Part model, mm, in its own coordinate system. A direction names the side the tool comes from. Round coordinates to 2 decimals unless told otherwise and drop trailing zeros. Loops run counter-clockwise (first coordinate to the right, second up) from the corner with the lowest first, then second, coordinate; pieces in that order, holes last.
from build123d import *

# Parameters (mm, degrees)
SKETCH_1_R      = 1
EXTRUDE_1_DEPTH = 1
SKETCH_1_3_W    = 1
SKETCH_1_3_H    = 4
EXTRUDE_2_DEPTH = 5
SKETCH_2_W      = 4
SKETCH_2_H      = 1
EXTRUDE_3_DEPTH = 2
FILLET_1_R      = 1
FILLET_2_R      = 2
FILLET_3_R      = 1


with BuildPart() as part:
    # 草圖1 → 填料-伸長1 (new body)
    with BuildSketch(Plane(origin=(0, 0, 0), x_dir=(1, 0, 0), z_dir=(0, 1, 0))):
        with BuildLine():
            ThreePointArc((0, -2), (2, 0), (0, 2))
            Line((0, 2), (-2, 2))
            Line((-2, 2), (-2, -2))
            Line((-2, -2), (0, -2))
        make_face()
        with Locations(Location((0, 0, 0), (0, 0, 270))):
            Circle(SKETCH_1_R, mode=Mode.SUBTRACT)
    extrude(amount=EXTRUDE_1_DEPTH)

    # 草圖1<3> → 填料-伸長2 (add)
    with BuildSketch(Plane(origin=(0, 0, 0), x_dir=(1, 0, 0), z_dir=(0, 1, 0))):
        with Locations((-2.5, 0)):
            Rectangle(SKETCH_1_3_W, SKETCH_1_3_H)
    extrude(amount=EXTRUDE_2_DEPTH)

    # 草圖2 → 填料-伸長3 (add)
    with BuildSketch(Plane(origin=(-2, 0, 0), x_dir=(0, 0, -1), z_dir=(1, 0, 0))):
        with Locations((0, 4.5)):
            Rectangle(SKETCH_2_W, SKETCH_2_H)
    extrude(amount=EXTRUDE_3_DEPTH)

    # 圓角1
    fillet_1_edges = [part.edges().sort_by_distance(p)[0] for p in [
        (0, 4.5, 2),
        (0, 4.5, -2),
    ]]
    fillet(fillet_1_edges, radius=FILLET_1_R)

    # 圓角2
    fillet_2_edges = [part.edges().sort_by_distance(p)[0] for p in [
        (-3, 0, 0),
    ]]
    fillet(fillet_2_edges, radius=FILLET_2_R)

    # 圓角3
    fillet_3_edges = [part.edges().sort_by_distance(p)[0] for p in [
        (-2, 1, 0),
    ]]
    fillet(fillet_3_edges, radius=FILLET_3_R - 0.0001)  # a hair under: the kernel refuses the full size


solid = part.part
1) Mould opens along X. For faces 4 (the face through (-0.301, 4.507, -1.715)), 5 (the face through (1.15, 0, -0.03)), 6 (the face through (-0.976, 0.493, -0.217)) say: released by +X, released by -X, zero draft, split by the parting line, or undercut.
Values:
face 4: released by +X
face 5: zero draft
face 6: undercut
2) Slice it at A-A, the plane z = 0.55. Give the cut face in (x, y).
Values:
outline: (-3, 2) arc R2 ccw to (-1, 0) - (-0.84, 0) - (-0.84, 1) - (-1, 1) arc R1 cw to (-2, 2) - (-2, 4) - (0, 4) - (0, 5) - (-3, 5) - close; (0.84, 0) - (1.92, 0) - (1.92, 1) - (0.84, 1) - close
3) Slice it at B-B, the plane y = 2.35. Give the cut face in (x, z).
Values:
outline: (-3, -2) - (-2, -2) - (-2, 2) - (-3, 2) - close
4) Slice it at D-D, the plane x = 1.15. Give the cut face in (y, z), then the cut area to 3 significant figures.
Values:
outline: (0, -1.64) - (1, -1.64) - (1, 1.64) - (0, 1.64) - close
area: 3.27 mm2
5) Wall check: line 1 along Y through (x, z) = (-0.15, 1.3); line 2 along Y through (x, z) = (0.1, 1.35); line 3 along X through (y, z) = (3.75, -1.05). Give the ranges that are in metal, low to high.
Values:
line 1: y = 0 to 1, 4 to 5
line 2: y = 0 to 1
line 3: x = -3 to -2
6) Drop flat-ended pins along their axis: pin 1 Ø3 at (x, y) = (-1.5, 3) entering from -Z; pin 2 Ø0.6 at (y, z) = (2.5, 1) entering from +X; pin 3 Ø1.1 at (y, z) = (4.5, 0) entering from +X. Give the stop position or say it passes through.
Values:
pin 1: stops at z = -2
pin 2: stops at x = -2
pin 3: stops at x = 0
7) Tool access for faces 1 (the face through (-1.699, 1.285, 0.028)), 2 (the face through (-0.301, 4.507, 1.715)), 3 (the face through (-3, 3, 0)): list every direction of +Z, -Z, +X, -X, +Y, -Y with a clear straight run to the whole face (end or side of a thin tool).
Values:
face 1: +Z, -Z, +X
face 2: +Z, +X, +Y
face 3: +Z, -Z, -X, +Y, -Y
8) Slice it at C-C, the plane z = -0.9. Give the cut face in (x, y), then the cut area to 3 significant figures.
Values:
outline: (-3, 2) arc R2 ccw to (-1, 0) - (-0.44, 0) - (-0.44, 1) - (-1, 1) arc R1 cw to (-2, 2) - (-2, 4) - (0, 4) - (0, 5) - (-3, 5) - close; (0.44, 0) - (1.79, 0) - (1.79, 1) - (0.44, 1) - close
area: 9.27 mm2
